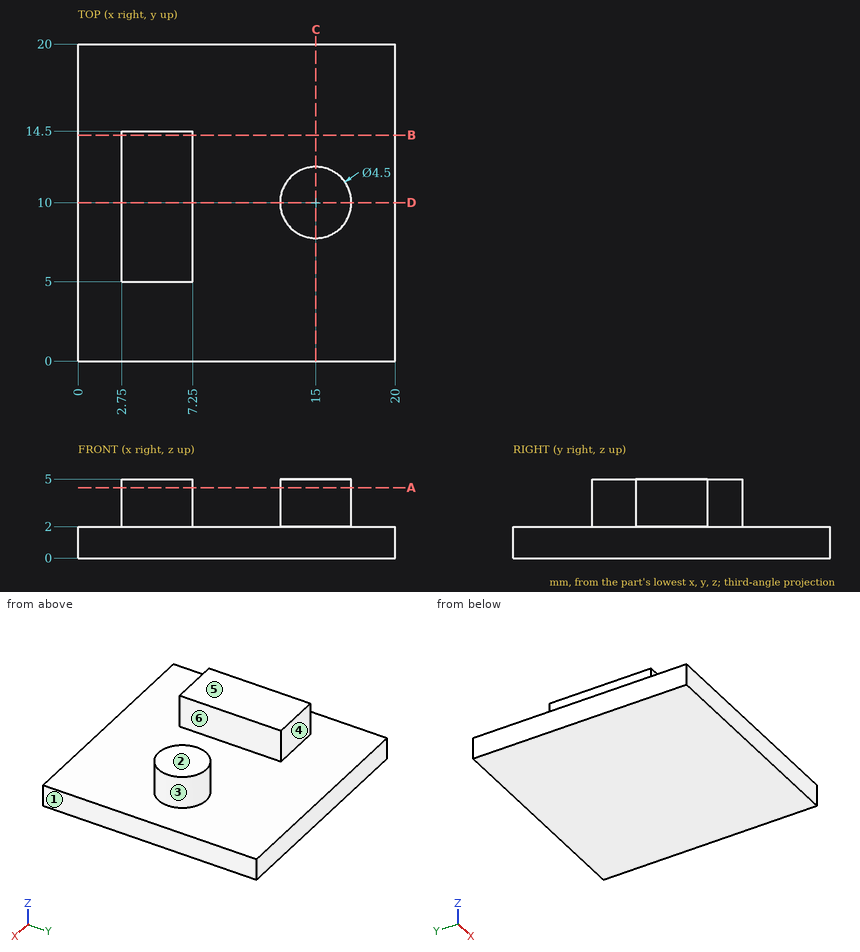
Input: dimensioned drawing with shaded views. Units: mm. Origin: part minimum x, y, z. A direction names the side the tool comes from. Coordinates: 2 decimals unless noted, no trailing zeros. Loops run counter-clockwise (first coordinate to the right, second up) from the corner with the lowest first, then second, coordinate; pieces in that order, holes last.
Q1. Section C-C, the plane x = 15. Return the cut outline in (y, z), and give its area (3 significant figures).
Results are:
outline: (0, 0) - (20, 0) - (20, 2) - (12.25, 2) - (12.25, 5) - (7.75, 5) - (7.75, 2) - (0, 2) - close
area: 53.5 mm2
Q2. Contact query for flat-ended pins moving along their axis: pin 1 (0.9 mm diameter, centred on y = 12, z = 4, fed in from -X); pin 2 (0.9 mm diameter, centred on x = 5, z = 4, fed in from -Y); pin 3 (2.5 mm diameter, centred on y = 7.5, z = 3.5, fed in from +X). Output: stop coordinate, or through.
Results are:
pin 1: stops at x = 2.75
pin 2: stops at y = 5
pin 3: stops at x = 16.87
Q3. Mould query, pull axis X, two halves, no side actions, for the marked faces 1, 2 and 3. Classes: +X half, -X half, draft (parallel to the pull), parting line (faces both ways), or undercut.
Results are:
face 1: +X half
face 2: draft
face 3: undercut
Q4. Section B-B, the plane y = 14.25. Return the cut outline in (x, z), and give its area (3 significant figures).
Results are:
outline: (0, 0) - (20, 0) - (20, 2) - (7.25, 2) - (7.25, 5) - (2.75, 5) - (2.75, 2) - (0, 2) - close
area: 53.5 mm2
Q5. Section D-D, the plane y = 10. Return the cut outline in (x, z).
Results are:
outline: (0, 0) - (20, 0) - (20, 2) - (17.25, 2) - (17.25, 5) - (12.75, 5) - (12.75, 2) - (7.25, 2) - (7.25, 5) - (2.75, 5) - (2.75, 2) - (0, 2) - close
Q6. Set-up query: the marked faces 4, 5 and 6. Return all of +Z, -Z, +X, -X, +Y, -Y with unobstructed straight access to the full face (end or side cutting, diameter ignored); none if empty.
Results are:
face 4: +Z, +X, -X, +Y
face 5: +Z, +X, -X, +Y, -Y
face 6: +Z, +Y, -Y
Q7. Section A-A, the plane z = 4.45. Return the cut outline in (x, y).
Results are:
outline: (2.75, 5) - (7.25, 5) - (7.25, 14.5) - (2.75, 14.5) - close; circle Ø4.5 at (15, 10)
Q8. Line query: line 1 along Z through (x, y) = (8.25, 12.25); line 2 along Y through (x, z) = (6.75, 3.3); line 3 along X through (y, z) = (5.25, 4.1). Output: solid intervals per line, ascending.
Results are:
line 1: z = 0 to 2
line 2: y = 5 to 14.5
line 3: x = 2.75 to 7.25
